Autodesk Inventor part; units mm, degrees
ref_plane "Plano inicial" through (0, 0, -21.3346) normal (0, 0, 1) x (1, 0, 0)
ref_plane "Plano final" through (0, 0, 2236.068) normal (0, 0, 1) x (1, 0, 0)
ref_plane "Plano de trabalho4" through (-28.0859, 9.362, -19.6589) normal (0.5248, -0.1749, -0.8331) x (-0.6498, 0.5499, -0.5248)
ref_plane "Plano inicial" through (0, 0, -21.3346) normal (0, 0, 1) x (1, 0, 0)
ref_plane "Plano final" through (0, 0, 2236.068) normal (0, 0, 1) x (1, 0, 0)
sketch "Esboço" plane through (0, 0, 0) normal (0, 0, 1) x (1, 0, 0)
  line L0 (-25.4, -15.875) -> (-25.4, 15.875)
  line L1 (-15.875, 25.4) -> (15.875, 25.4)
  line L2 (25.4, 15.875) -> (25.4, -15.875)
  line L3 (15.875, -25.4) -> (-15.875, -25.4)
  arc A0 (-25.4, -15.875) -> (-15.875, -25.4) centre (-15.875, -15.875) ccw
  arc A1 (-15.875, 25.4) -> (-25.4, 15.875) centre (-15.875, 15.875) ccw
  arc A2 (25.4, 15.875) -> (15.875, 25.4) centre (15.875, 15.875) ccw
  arc A3 (15.875, -25.4) -> (25.4, -15.875) centre (15.875, -15.875) ccw
  arc A4 (-15.875, 20.6375) -> (-20.6375, 15.875) centre (-15.875, 15.875) ccw
  line L4 (-15.875, 20.6375) -> (15.875, 20.6375)
  arc A5 (20.6375, 15.875) -> (15.875, 20.6375) centre (15.875, 15.875) ccw
  line L5 (20.6375, 15.875) -> (20.6375, -15.875)
  arc A6 (15.875, -20.6375) -> (20.6375, -15.875) centre (15.875, -15.875) ccw
  line L6 (15.875, -20.6375) -> (-15.875, -20.6375)
  arc A7 (-20.6375, -15.875) -> (-15.875, -20.6375) centre (-15.875, -15.875) ccw
  line L7 (-20.6375, -15.875) -> (-20.6375, 15.875)
  line L8 (0, 38.3218) -> (0, -38.3218) construction
  line L9 (-38.3218, 0) -> (38.3218, 0) construction
  dimension "d10" = 50.8
  dimension "d11" = 50.8
  dimension "d12" = 4.7625
  dimension "d15" = 25.4
  dimension "d16" = 25.4
  dimension "d17" = 9.525
extrude "Corpo" add sketch "Esboço" along normal up to surface (2257.4026 mm away) from surface at -21.3346
sketch "Sketch3" plane through (0, 0, 0) normal (0, 0, 1) x (1, 0, 0)
  line L0 (0, 0) -> (10, 0)
ref_plane "Work Plane3" through (0, 0, 0) normal (0, -1, 0) x (1, 0, 0)
sketch "Sketch4" plane through (0, 0, 0) normal (0, -1, 0) x (1, 0, 0)
  line L0 (-2, -21.3346) -> (12, -21.3346)
  line L1 (-2, 2236.068) -> (12, 2236.068)
  dimension "d19" = 2257.4026
ref_plane "Plano de trabalho4" through (-28.0859, 9.362, -19.6589) normal (0.5248, -0.1749, -0.8331) x (-0.6498, 0.5499, -0.5248)
split "Dividir1" plane through (-28.0859, 9.362, -19.6589) removes the side toward (0.5248, -0.1749, -0.8331)
equation "\"d10\" = G_H"
equation "\"d11\" = G_W"
equation "\"d12\" = G_T"
equation "\"d15\" = 0.5 * d10"
equation "\"d16\" = 0.5 * d11"
equation "\"d17\" = G_IR"
equation "\"d3\" = G_L"
equation "\"G_W\" = 50.8"
equation "\"G_H\" = 50.8"
equation "\"G_T\" = 4.7625"
equation "\"G_IR\" = 9.525"
equation "\"G_L\" = 2255.40246"
equation "\"G_OFFSET_START\" = 21.3346"
equation "\"G_OFFSET_END\" = 0"
equation "\"d13\" = -G_OFFSET_START"
equation "\"d14\" = G_OFFSET_END + B_L"
equation "\"B_L\" = 2236.06798"
properties part number "AISC - 2 x 2 x 3/16 - 88,795" material "Aço, suave"
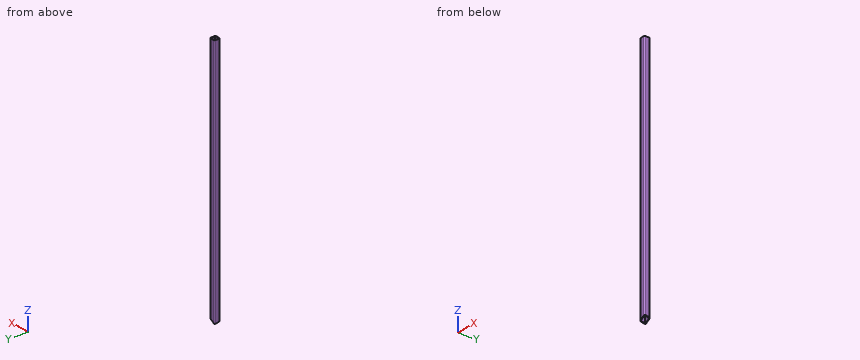
The model under review builds one solid part; all positions refer to its coordinate system, in mm. Round coordinates to 2 decimals unless told otherwise and drop trailing zeros. Loops run counter-clockwise (first coordinate to the right, second up) from the corner with the lowest first, then second, coordinate; pieces in that order, holes last. Notation, with made-up numbers: (-31, 47.5) -> (18, 47.5) arc R26 cw to (18, 79.5) -> close; hole circle Ø7 at (31.25, 9). An arc over 180 degrees is marked (long way). Answer as CSV lines item,"result".
1) Add section C-C on y = -4.5. Write out the cut boundary in (x, z), plus the area to 3 significant figures.
Geometry results:
outline,"(-25.4, -15.06) -> (-20.64, -12.06) -> (-20.64, 2236.07) -> (-25.4, 2236.07) -> close; (20.64, 13.94) -> (25.4, 16.94) -> (25.4, 2236.07) -> (20.64, 2236.07) -> close"
area,"21,300 mm²"
2) To check wall thickness, follow line 1 along X through (y, z) = (11.5, 256.5); line 2 along Y through (x, z) = (17, 1875). State the ranges of each line that lie inside material, in increasing order. Write a range as from..to.
Geometry results:
line 1,"x = -25.4..-20.64, 20.64..25.4"
line 2,"y = -25.33..-20.5, 20.5..25.33"
3) Add section B-B on x = -7.5. Write out the cut boundary in (y, z), plus the area to 3 significant figures.
Geometry results:
outline,"(-25.4, 0.61) -> (-20.64, -0.39) -> (-20.64, 2236.07) -> (-25.4, 2236.07) -> close; (20.64, -9.06) -> (25.4, -10.06) -> (25.4, 2236.07) -> (20.64, 2236.07) -> close"
area,"21,300 mm²"
4) For P1, Ø4, axis at x = 18.5, y = 7.5, coming from the -Z side, flat-tipped, find the tip position at first contact; note if it passes through.
Geometry results:
P1,"passes through"
